Job drawing, mm, ordinate dimensions from the low corner. One solid piece. A direction names the side the tool comes from. Coordinates: 2 decimals unless noted, no trailing zeros. Write each loop counter-clockwise with the first axis right and the second up, starting at its lowest first coordinate (ties: lowest second). Pieces come first, ordered by that corner, then holes.
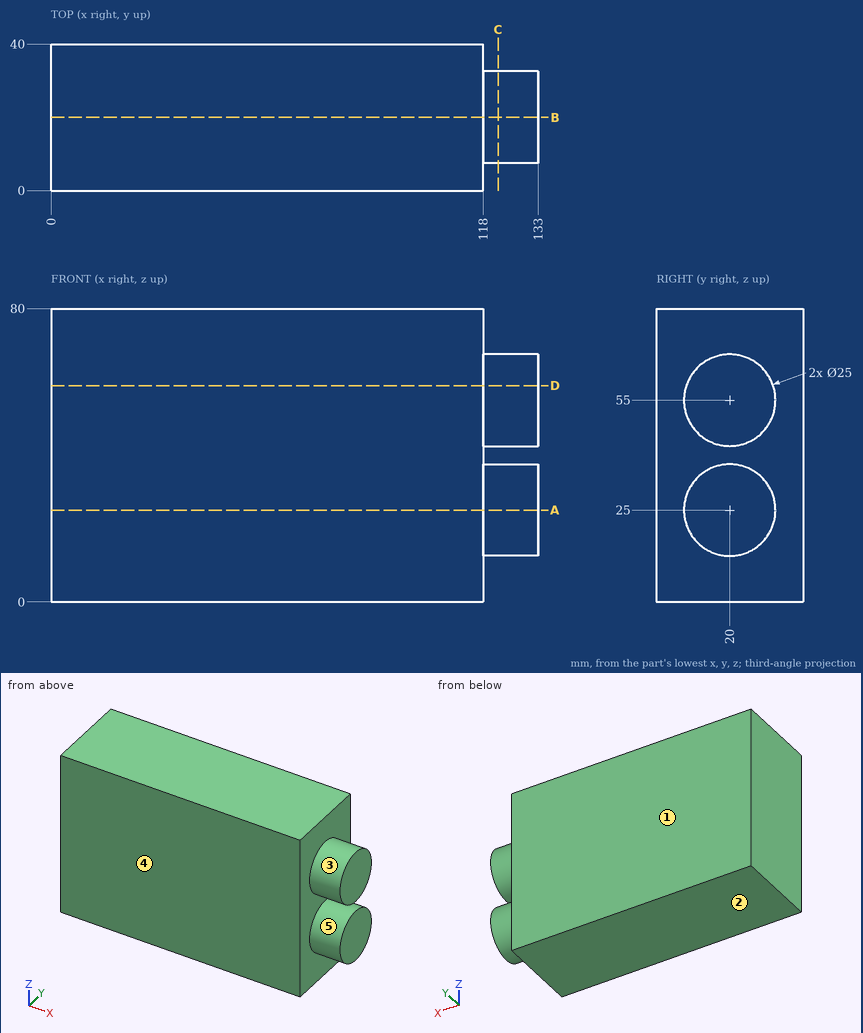
1. 3-axis set-ups, long thin cutter, end or side, ignore diameter. For the marked faces 4 and 5: which of +Z, -Z, +X, -X, +Y, -Y reach the whole face in a straight line?
Computed values:
face 4: +Z, -Z, +X, -X, -Y
face 5: +X
2. Saw through at A-A on z = 25. List the corners of the cut face in (x, y).
Computed values:
outline: (0, 0) - (118, 0) - (118, 7.5) - (133, 7.5) - (133, 32.5) - (118, 32.5) - (118, 40) - (0, 40) - close
3. Mould opens along Z. For the marked faces 1, 2 and 3 say: +Z half, -Z half, draft (parallel to the pull), parting line (faces both ways), or undercut.
Computed values:
face 1: draft
face 2: -Z half
face 3: undercut
4. Saw through at C-C on x = 122. List the corners of the cut face in (y, z), plus the area to 3 significant figures.
Computed values:
outline: circle Ø25 at (20, 25); circle Ø25 at (20, 55)
area: 982 mm2
5. Saw through at D-D on z = 59. List the corners of the cut face in (x, y).
Computed values:
outline: (0, 0) - (118, 0) - (118, 8.16) - (133, 8.16) - (133, 31.84) - (118, 31.84) - (118, 40) - (0, 40) - close
6. Probe line 1 along X through (y, z) = (9.5, 69.5); line 2 along Z through (x, y) = (123, 30.5). List the from-to ranges inside material, lowest first.
Computed values:
line 1: x = 0 to 118
line 2: z = 18.22 to 31.78, 48.22 to 61.78
7. Saw through at B-B on y = 20. List the corners of the cut face in (x, z), plus the area to 3 significant figures.
Computed values:
outline: (0, 0) - (118, 0) - (118, 12.5) - (133, 12.5) - (133, 37.5) - (118, 37.5) - (118, 42.5) - (133, 42.5) - (133, 67.5) - (118, 67.5) - (118, 80) - (0, 80) - close
area: 10,200 mm2
